from build123d import *

# Parameters (mm, degrees)
BOSS_EXTRUDE1_DEPTH      = 55
BOSS_EXTRUDE2_DEPTH      = 10
BOSS_EXTRUDE2_DEPTH_BACK = 65
SKETCH2_R                = 55
SKETCH3_R                = 7.522289104
CUT_EXTRUDE1_DEPTH       = 1000.987090528


with BuildPart() as part:
    # Sketch1 → Boss-Extrude1 (new body)
    with BuildSketch(Plane(origin=(0, 0, 0), x_dir=(1, 0, 0), z_dir=(0, 1, 0))):
        with BuildLine():
            Line((0, -140.97167407), (0, 921.782563534))
            Line((0, 921.782563534), (-98.380397364, 921.782563534))
            Line((-98.380397364, 921.782563534), (-123.405755698, 28.326097488))
            ThreePointArc((-123.405755698, 28.326097488), (-125.417562899, -114.522053174), (-98.380397364, -254.80260491))
            Line((-98.380397364, -254.80260491), (108.641172319, -548.724400702))
            Line((108.641172319, -548.724400702), (189.500983305, -474.147655215))
            Line((189.500983305, -474.147655215), (123.733893044, -401.532470648))
            ThreePointArc((123.733893044, -401.532470648), (42.669425171, -280.368501556), (0, -140.97167407))
        make_face()
    extrude(amount=BOSS_EXTRUDE1_DEPTH)

    # Sketch2 → Boss-Extrude2 (add, two sides: drawn at the far end of the back side and taken through both)
    with BuildSketch(Plane(origin=(0, 55, 0), x_dir=(1, 0, 0), z_dir=(0, 1, 0)).offset(-BOSS_EXTRUDE2_DEPTH_BACK)):
        with Locations(Location((149.071077812, -511.436027959, 0), (0, 0, 270))):
            Circle(SKETCH2_R)
        with Locations(Location((-49.190198682, 921.782563534, 0), (0, 0, 270))):
            Circle(SKETCH2_R)
    extrude(amount=BOSS_EXTRUDE2_DEPTH + BOSS_EXTRUDE2_DEPTH_BACK)

    # Sketch3 → Cut-Extrude1 (cut, through all)
    with BuildSketch(Plane(origin=(0, 55, 0), x_dir=(1, 0, 0), z_dir=(0, 1, 0))):
        with Locations(Location((-54.735242724, 30.764070808, 0), (0, 0, 270))):
            Circle(SKETCH3_R)
        with Locations(Location((-62.623286792, -113.195627247, 0), (0, 0, 270))):
            Circle(SKETCH3_R)
    extrude(amount=-CUT_EXTRUDE1_DEPTH, mode=Mode.SUBTRACT)


solid = part.part
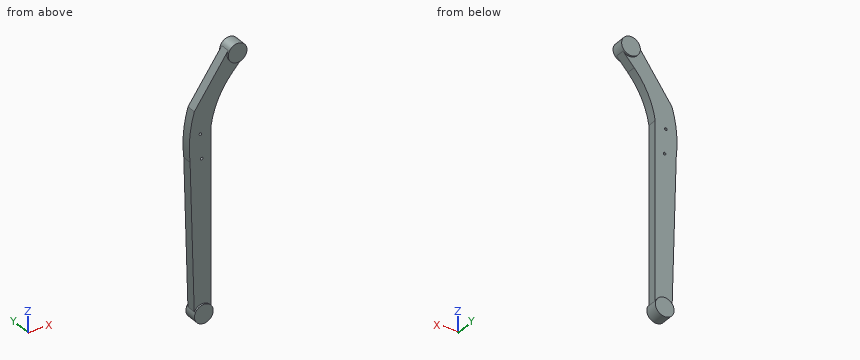
Check sheet for the modelled part. Datum: model origin and axes. Units: mm. Give positions to 0.01 mm unless a question says otherwise; leave off trailing zeros. Write each loop counter-clockwise with the first axis right and the second up, starting at its lowest first coordinate (ties: lowest second). Pieces come first, ordered by that corner, then holes. Notation, with made-up numbers: (76, -8) -> (116, -8) arc R26 ccw to (116, 22) -> close; hole circle Ø4 at (34, 29.5). An arc over 180 degrees is marked (long way). Write item = value, one per line.
Item 1: Sectioned sample at B-B on x = 56. Record the boundary of the cut face in (y, z).
Output:
outline = (0, 306.44) -> (55, 306.44) -> (55, 473.99) -> (0, 473.99) -> close
Item 2: Sectioned sample at C-C on z = 14. Record the boundary of the cut face in (x, y), and give its area (3 significant figures).
Output:
outline = (-127.05, 0) -> (0, 0) -> (0, 55) -> (-127.05, 55) -> close
area = 6,990 mm^2
Item 3: Sectioned sample at A-A on y = 28. Record the boundary of the cut face in (x, z), and give its area (3 significant figures).
Output:
outline = (-123.41, -28.33) -> (-99.03, -898.53) arc R55 ccw (long way) to (0, -897.18) -> (0, 140.97) arc R500 cw to (123.73, 401.53) -> (189.5, 474.15) arc R55 ccw (long way) to (100.34, 536.94) -> (-98.38, 254.8) arc R699.87 ccw to start; hole circle Ø15.04 at (-62.62, 113.2); hole circle Ø15.04 at (-54.74, -30.76)
area = 176,000 mm^2
Item 4: Gauge pin test, flat ends, axial feed: pin 1 (10 mm diameter, centred on y = 18, z = -105, fed in from +X); pin 2 (10 mm diameter, centred on y = 16, z = 398.5, fed in from +X); pin 3 (10 mm diameter, centred on x = 54.5, z = 336.5, fed in from +Y). Record the tip position at first contact, or that the pin passes through.
Output:
pin_1 = 0
pin_2 = 125.52
pin_3 = 55
Item 5: Scan lines: probe 1 along Z at (x, y) = (-61.5, 26.5); probe 2 along Y at (x, z) = (110, 462.5); probe 3 along Z at (x, y) = (149, -4.5). Record each from-to range of solid material in increasing order. Write a range as from..to.
Output:
probe_1 = -975.39..-34.05, -27.47..105.76, 120.63..307.16
probe_2 = 0..55
probe_3 = 456.44..566.44
